Geometry check sheet. Reference: the model listing, model coordinates, mm. Face numbers are marked on the shaded views. A direction names the side the tool comes from. Coordinates: 2 decimals unless noted, no trailing zeros. Write each loop counter-clockwise with the first axis right and the second up, starting at its lowest first coordinate (ties: lowest second). Pieces come first, ordered by that corner, then holes. Notation, with made-up numbers: (-3, 53.5) -> (41, 53.5) arc R20 cw to (41, 92.5) -> close; hole circle Ø4 at (49.5, -36.5). An arc over 180 degrees is marked (long way). Use a Markdown table: item, result.
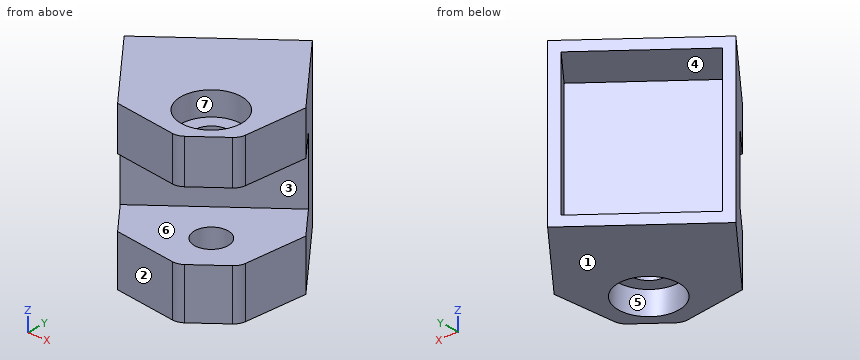
```python
from build123d import *

# Parameters (mm, degrees)
CYLINDER025_R          = 2.5
CYLINDER025_DEPTH      = 32
CYLINDER027_R          = 4.5
CYLINDER027_DEPTH      = 5
CYLINDER026_R          = 4.5
CYLINDER026_DEPTH      = 5
BOX007_W               = 24
BOX007_H               = 14
BOX007_DEPTH           = 10
BOX005_W               = 18
BOX005_H               = 10
BOX005_DEPTH           = 21
BOX006_W               = 21
BOX006_H               = 22
BOX006_DEPTH           = 24
CHAMFER_SIZE           = 7
FILLET_R               = 2
CUT022_PLACEMENT_ANGLE = 39


with BuildPart() as cylinder025:
    # Cylinder025 → Cylinder025 (new body)
    with BuildSketch(Plane(origin=(55, -39, -20), x_dir=(1, 0, 0), z_dir=(0, 0, 1))):
        Circle(CYLINDER025_R)
    extrude(amount=CYLINDER025_DEPTH)


with BuildPart() as cylinder027:
    # Cylinder027 → Cylinder027 (new body)
    with BuildSketch(Plane(origin=(55, -39, 8), x_dir=(1, 0, 0), z_dir=(0, 0, 1))):
        Circle(CYLINDER027_R)
    extrude(amount=CYLINDER027_DEPTH)


with BuildPart() as cylinder026:
    # Cylinder026 → Cylinder026 (new body)
    with BuildSketch(Plane(origin=(55, -39, -14), x_dir=(1, 0, 0), z_dir=(0, 0, 1))):
        Circle(CYLINDER026_R)
    extrude(amount=CYLINDER026_DEPTH)


with BuildPart() as box007:
    # Box007 → Box007 (new body)
    with BuildSketch(Plane(origin=(43, -46, -5), x_dir=(1, 0, 0), z_dir=(0, 0, 1))):
        with Locations((12, 7)):
            Rectangle(BOX007_W, BOX007_H)
    extrude(amount=BOX007_DEPTH)


with BuildPart() as box005:
    # Box005 → Box005 (new body)
    with BuildSketch(Plane(origin=(46, -30, -11), x_dir=(1, 0, 0), z_dir=(0, 0, 1))):
        with Locations((9, 5)):
            Rectangle(BOX005_W, BOX005_H)
    extrude(amount=BOX005_DEPTH)


with BuildPart() as cut022:
    # Box006 → Box006 (new body)
    with BuildSketch(Plane(origin=(44.5, -45, -12.5), x_dir=(1, 0, 0), z_dir=(0, 0, 1))):
        with Locations((10.5, 11)):
            Rectangle(BOX006_W, BOX006_H)
    extrude(amount=BOX006_DEPTH)

    # Cut018: cut Box005
    add(box005.part, mode=Mode.SUBTRACT)

    # Chamfer
    chamfer_edges = [cut022.edges().sort_by_distance(p)[0] for p in [
        (44.5, -45, -0.5),
        (65.5, -45, -0.5),
    ]]
    chamfer(chamfer_edges, length=CHAMFER_SIZE)

    # Fillet
    fillet_edges = [cut022.edges().sort_by_distance(p)[0] for p in [
        (51.5, -45, -0.5),
        (58.5, -45, -0.5),
    ]]
    fillet(fillet_edges, radius=FILLET_R)

    # Cut019: cut Box007
    add(box007.part, mode=Mode.SUBTRACT)

    # Cut020: cut Cylinder026
    add(cylinder026.part, mode=Mode.SUBTRACT)

    # Cut021: cut Cylinder027
    add(cylinder027.part, mode=Mode.SUBTRACT)

    # Cut022: cut Cylinder025
    add(cylinder025.part, mode=Mode.SUBTRACT)


with BuildPart() as cut022_1:
    # Cut022 placement: moved
    add(cut022.part.moved(Location((-40, -38, 0))).rotate(Axis((-40, -38, 0), (0, 0, 1)), CUT022_PLACEMENT_ANGLE))


solid = cut022_1.part
```
Item 1: Tool access check on the marked faces 5, 6 and 7. Record the directions out of +Z, -Z, +X, -X, +Y, -Y that give a thin tool (end or side, any length) a straight path to the whole face; none if there is none.
Answer block:
| item | result |
|---|---|
| face 5 | -Z |
| face 6 | +X, -Y |
| face 7 | +Z |
Item 2: Depth check by flat-ended pin: P1, Ø1.5, axis at y = -30.5, z = 7.5, coming from the -X side; P2, Ø1.5, axis at y = -23, z = -8, coming from the +X side; P3, Ø7, axis at x = 27.29, y = -33.7, coming from the +Z side. Enter the tip coordinate at first touch or a pass-through.
Answer block:
| item | result |
|---|---|
| P1 | stops at x = 10.58 |
| P2 | stops at x = 32.74 |
| P3 | stops at z = 8 |
Item 3: Section check A-A on y = -32.75. Record the boundary of the cut face in (x, z), then the cut area to 3 significant figures.
Answer block:
| item | result |
|---|---|
| outline | (13.01, -12.5) -> (22.89, -12.5) -> (22.89, -9) -> (24.97, -9) -> (24.97, -5) -> (17.33, -5) -> (17.33, 5) -> (24.97, 5) -> (24.97, 8) -> (22.89, 8) -> (22.89, 11.5) -> (13.01, 11.5) -> close; (29.6, -9) -> (31.69, -9) -> (31.69, -12.5) -> (34.14, -12.5) -> (34.14, -5) -> (29.6, -5) -> close; (29.6, 5) -> (34.14, 5) -> (34.14, 11.5) -> (31.69, 11.5) -> (31.69, 8) -> (29.6, 8) -> close |
| area | 245 mm^2 |
Item 4: Section check B-B on z = 4. Record the boundary of the cut face in (x, y).
Answer block:
| item | result |
|---|---|
| outline | (9.06, -27.87) -> (14.72, -34.86) -> (31.04, -21.65) -> (25.38, -14.65) -> (24.21, -15.6) -> (28.62, -21.04) -> (14.63, -32.37) -> (10.22, -26.93) -> close |
Item 5: Mould release check, pull along Z, two halves, no side actions. Record for the marked faces 1, 2, 3 and 4: +Z half, -Z half, draft (parallel to the pull), parting line (faces both ways), or undercut.
Answer block:
| item | result |
|---|---|
| face 1 | -Z half |
| face 2 | draft |
| face 3 | undercut |
| face 4 | undercut |
Item 6: Section check C-C on y = -37.25. Record the boundary of the cut face in (x, z).
Answer block:
| item | result |
|---|---|
| outline | (16.65, -12.5) -> (24.53, -12.5) -> (24.53, -9) -> (30.05, -9) -> (30.05, -12.5) -> (32.43, -12.5) -> (32.43, -5) -> (16.65, -5) -> close; (16.65, 5) -> (32.43, 5) -> (32.43, 11.5) -> (30.05, 11.5) -> (30.05, 8) -> (24.53, 8) -> (24.53, 11.5) -> (16.65, 11.5) -> close |
Item 7: Section check D-D on z = 7. Record the boundary of the cut face in (x, y), then the cut area to 3 significant figures.
Answer block:
| item | result |
|---|---|
| outline | (9.06, -27.87) -> (18.5, -39.53) -> (27.52, -40.47) arc R2 ccw to (28.99, -40.04) -> (33.14, -36.68) arc R2 ccw to (33.87, -35.33) -> (34.82, -26.31) -> (25.38, -14.65) -> (24.21, -15.6) -> (28.62, -21.04) -> (14.63, -32.37) -> (10.22, -26.93) -> close; hole circle Ø5 at (27.29, -33.7) |
| area | 267 mm^2 |
Item 8: Thickness scan on L1, parallel to Z at x = 16, y = -26; L2, parallel to Z at x = 29.75, y = -29.25; L3, parallel to X at y = -31.5, z = 10.5. Record the ranges inside material, lowest first. Write a range as [from, to].
Answer block:
| item | result |
|---|---|
| L1 | z = [-12.5, -11], [10, 11.5] |
| L2 | z = [-12.5, -5], [5, 11.5] |
| L3 | x = [12, 23.36], [31.21, 34.27] |
